The drawing under review shows one solid part. Ordinate dimensions are in mm from its lowest x, y, z. A direction names the side the tool comes from. Coordinates: 2 decimals unless noted, no trailing zeros. Order: outer loops, then holes, each group sorted by start corner. A loop starts at its lowest first (then second) coordinate and runs counter-clockwise, first axis right, second up. Notation, with made-up numbers: (29, 15.25) -> (70, 15.25) arc R33 cw to (70, 44.25) -> close; hole circle Ø2 at (-29, 86). An arc over 180 degrees is marked (long way). Use a Markdown table: item, result. Add a question column.
Q1. Add section D-D (x = 21.5). State the section outline as (y, z) points.
Q2. Insertion check: pin 1 (4.5 mm diameter, centred on y = 76.2, z = 25.4, fed in from +X). The pin has a flat end and moves straight along its axis. Give the tip position at first contact, or say it passes through.
Q3. Wall thickness on probe 1 along Y at (x, z) = (12.7, 0.4); probe 2 along X at (y, z) = (6.5, 39); probe 3 along Y at (x, z) = (24.4, 25.4): over which ranges is each line inside the solid? List them lowest first.
Q4. Add section A-A (x = 12.7). Count the separate pieces of the cut face and the enclosed holes in it.
Q5. The part is to be moulded in two halves that separate along Z. For the marked faces 3, 4, 5 and 6, say which applies: pulls with the +Z half, pulls with the -Z half, needs draft (parallel to the pull), parting line crosses it, or undercut.
Q6. Machinability: for the marked faces 1 and 2, which of the approach directions +Z, -Z, +X, -X, +Y, -Y give a long, thin tool a straight path to every point of the face, cutting with its end or side? Answer none if there is none.
Q7. Add section C-C (y = 80). State the section outline as (x, z) points.
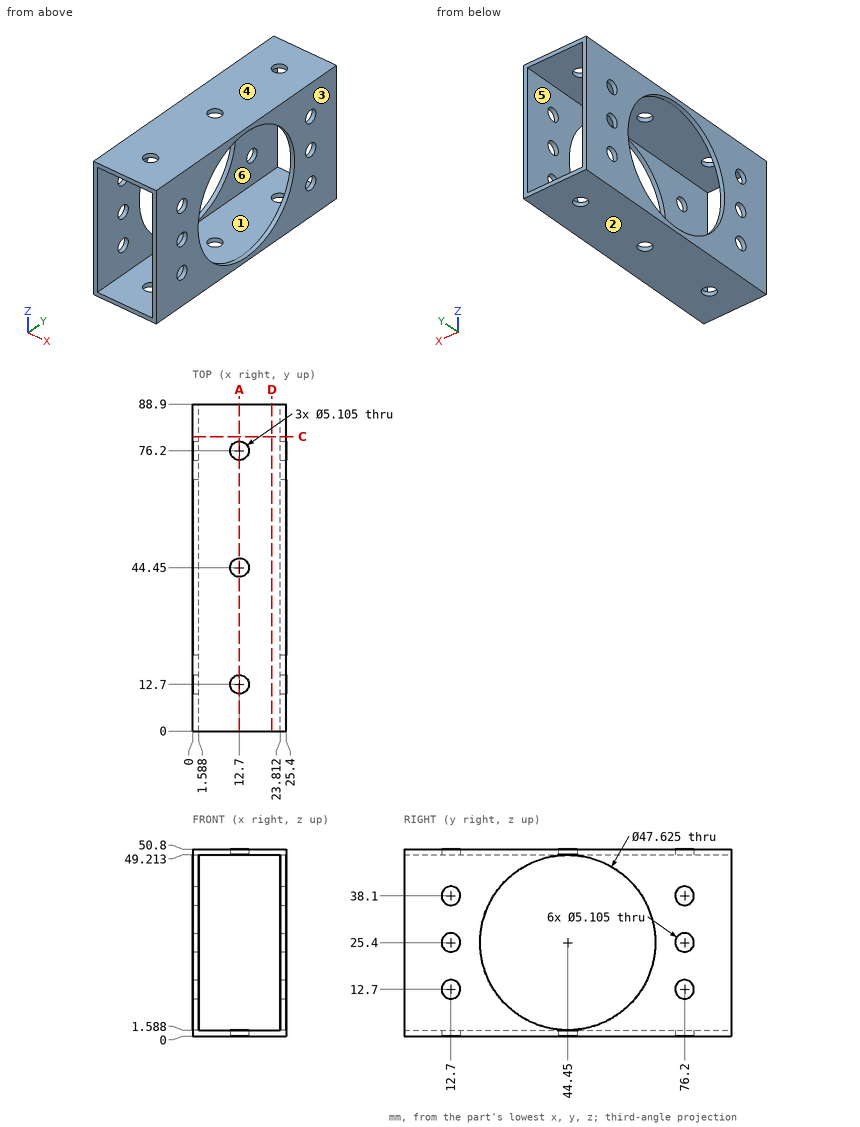
Established:
| question | item | result |
|---|---|---|
| 1 | outline | (0, 0) -> (88.9, 0) -> (88.9, 1.59) -> (0, 1.59) -> close; (0, 49.21) -> (88.9, 49.21) -> (88.9, 50.8) -> (0, 50.8) -> close |
| 2 | pin 1 | through |
| 3 | probe 1 | 0 to 10.15, 15.25 to 41.9, 47 to 73.65, 78.75 to 88.9 |
| 3 | probe 2 | 0 to 1.59, 23.81 to 25.4 |
| 3 | probe 3 | 0 to 10.15, 15.25 to 20.64, 68.26 to 73.65, 78.75 to 88.9 |
| 4 | separate pieces | 8 |
| 4 | enclosed holes | 0 |
| 5 | face 3 | needs draft |
| 5 | face 4 | pulls with the +Z half |
| 5 | face 5 | undercut |
| 5 | face 6 | undercut |
| 6 | face 1 | +Y, -Y |
| 6 | face 2 | -Z, +X, -X, +Y, -Y |
| 7 | outline | (0, 0) -> (25.4, 0) -> (25.4, 50.8) -> (0, 50.8) -> close; hole (1.59, 1.59) -> (23.81, 1.59) -> (23.81, 49.21) -> (1.59, 49.21) -> close |
